For this review, take the finished solid that the model builds, in its own axes (mm). Face numbers are marked on the shaded views. Give positions to 0.01 mm unless a question says otherwise; leave off trailing zeros. Order: outer loops, then holes, each group sorted by start corner. A loop starts at its lowest first (then second) coordinate and runs counter-clockwise, first axis right, second up. Notation, with made-up numbers: M -20.5,34 L 10.5,34 A16 ccw 10.5,42 Z; hole C -2,27.5 d5. An arc over 180 degrees is marked long. Answer as CSV lines item,"result". Start each with the question number.
1. For line 1 along X through (y, z) = (10.9, 0); line 2 along X through (y, z) = (1.6, 0); line 3 along Y through (x, z) = (-49, 4.75), list the stretches that pass through material, from the lowest coordinate up.
2. Mouldability with a two-part tool opening along Y and no side actions: class the marked faces 1, 2 and 3 as pulls with the +Y half, pulls with the -Y half, needs draft (parallel to the pull), parting line crosses it, or undercut.
3. We need section B-B, the plane x = -50.5. Give the boundary of the cut face in (y, z).
4. We need section A-A, the plane x = -3. Give the boundary of the cut face in (y, z).
5. We need section C-C, the plane x = -17.5. Give the boundary of the cut face in (y, z).
6. Clearance check with flat-ended pins moving along their axes: P1, Ø5, axis at x = -26, y = 11.5, coming from the +Z side; P2, Ø1.2, axis at x = 2.5, z = 0, coming from the -Y side; P3, Ø12, axis at x = -38, y = 7, coming from the -Z side. State where each tip first meets the part, or that it passes through.
from build123d import *

# Parameters (mm, degrees)
BOSS_EXTRUDE1_DEPTH = 14.11
SKETCH2_R           = 5.95
CUT_EXTRUDE1_DEPTH  = 5.6
SKETCH3_R           = 6.9
CUT_EXTRUDE2_DEPTH  = 0.6
SKETCH4_R           = 2.5
CUT_EXTRUDE3_DEPTH  = 70.144106761
SKETCH5_R           = 0.9
CUT_EXTRUDE4_DEPTH  = 4.4
SKETCH6_R           = 6
CUT_EXTRUDE6_DEPTH  = 2.5
BOSS_EXTRUDE5_DEPTH = 0.4
BOSS_EXTRUDE6_REACH = 73.866
SKETCH13_RX         = 6
SKETCH13_RY         = 4.596266659
SKETCH14_R          = 2.5
CUT_EXTRUDE8_DEPTH  = 8


with BuildPart() as part:
    # Sketch1 → Boss-Extrude1 (new body)
    with BuildSketch(Plane(origin=(0, 0, 0), x_dir=(1, 0, 0), z_dir=(0, 1, 0))):
        with BuildLine():
            Line((-62.34882326, 5.996720639), (-1.914938962, 7.995627519))
            ThreePointArc((-1.914938962, 7.995627519), (6.349523848, 0), (-1.914938962, -7.995627519))
            Line((-1.914938962, -7.995627519), (-62.34882326, -5.996720639))
            ThreePointArc((-62.34882326, -5.996720639), (-68.150476152, 0), (-62.34882326, 5.996720639))
        make_face()
    extrude(amount=BOSS_EXTRUDE1_DEPTH)

    # Sketch2 → Cut-Extrude1 (cut)
    with BuildSketch(Plane(origin=(0, 14.11, 0), x_dir=(1, 0, 0), z_dir=(0, 1, 0))):
        with Locations(Location((-1.650476152, 0, 0), (0, 0, 270))):
            Circle(SKETCH2_R)
    extrude(amount=-CUT_EXTRUDE1_DEPTH, mode=Mode.SUBTRACT)

    # Sketch3 → Cut-Extrude2 (cut)
    with BuildSketch(Plane(origin=(0, 14.11, 0), x_dir=(1, 0, 0), z_dir=(0, 1, 0))):
        with Locations(Location((-1.650476152, 0, 0), (0, 0, 270))):
            Circle(SKETCH3_R)
    extrude(amount=-CUT_EXTRUDE2_DEPTH, mode=Mode.SUBTRACT)

    # Sketch4 → Cut-Extrude3 (cut, through all)
    with BuildSketch(Plane(origin=(0, 8.51, 0), x_dir=(1, 0, 0), z_dir=(0, 1, 0))):
        with Locations(Location((-1.650476152, 0, 0), (0, 0, 270))):
            Circle(SKETCH4_R)
    extrude(amount=-CUT_EXTRUDE3_DEPTH, mode=Mode.SUBTRACT)

    # Sketch5 → Cut-Extrude4 (cut)
    with BuildSketch(Plane(origin=(0, 8.51, 0), x_dir=(1, 0, 0), z_dir=(0, 1, 0))):
        with Locations(Location((-4.832456668, 3.181980515, 0), (0, 0, 270))):
            Circle(SKETCH5_R)
    extrude(amount=-CUT_EXTRUDE4_DEPTH, mode=Mode.SUBTRACT)

    # Sketch6 → Cut-Extrude6 (cut)
    with BuildSketch(Plane.XZ):
        with Locations(Location((-1.650476152, 0, 0), (0, 0, 270))):
            Circle(SKETCH6_R)
    extrude(amount=-CUT_EXTRUDE6_DEPTH, mode=Mode.SUBTRACT)

    # Sketch10 → Boss-Extrude5 (add)
    with BuildSketch(Plane.XZ.offset(-2.5)):
        with BuildLine():
            Line((0.75768614, -0.671382434), (4.34720185, -0.1669089))
            ThreePointArc((4.34720185, -0.1669089), (4.29113226, 0.835038606), (4.068855648, 1.813627238))
            Line((4.068855648, 1.813627238), (0.479339938, 1.309153704))
            ThreePointArc((0.479339938, 1.309153704), (0.82519402, 0.347932752), (0.75768614, -0.671382434))
        make_face()
        with BuildLine():
            Line((-7.648154155, 0.1669089), (-4.058638445, 0.671382434))
            ThreePointArc((-4.058638445, 0.671382434), (-4.126146324, -0.347932752), (-3.780292243, -1.309153704))
            Line((-3.780292243, -1.309153704), (-7.369807953, -1.813627238))
            ThreePointArc((-7.369807953, -1.813627238), (-7.592084565, -0.835038606), (-7.648154155, 0.1669089))
        make_face()
    extrude(amount=BOSS_EXTRUDE5_DEPTH)

    # Boss-Extrude6: up to this plane
    boss_extrude6_end = Plane(origin=(-1.650476152, 14.11, 0), z_dir=(0, 1, 0))
    # Sketch13 → Boss-Extrude6 (add, up to the surface)
    with BuildSketch(Plane(origin=(-0.382193209, 13.778273936, -11.555025608), x_dir=(0.9997443283307086, 0.02124917717972034, -0.007729840862870826), z_dir=(-0.02124917717972034, 0.766044443118977, -0.6424362876081342)), mode=Mode.PRIVATE) as boss_extrude6_sk1:
        with Locations(Location((-61.834760146, -9.545189308), (0, 0, -178.105579493))):
            Ellipse(SKETCH13_RX, SKETCH13_RY)
    boss_extrude6_tool1 = split(extrude(boss_extrude6_sk1.sketch, amount=-BOSS_EXTRUDE6_REACH, mode=Mode.PRIVATE), bisect_by=boss_extrude6_end, keep=Keep.BOTH, mode=Mode.PRIVATE)
    add(boss_extrude6_tool1.solids().sort_by_distance((-62.274927, 18.596512, -3.762573))[0])

    # Sketch14 → Cut-Extrude8 (cut)
    with BuildSketch(Plane(origin=(-0.382193209, 13.778273936, -11.555025608), x_dir=(0.9997742107441985, 0.01628149028495012, -0.013654325502060603), z_dir=(-0.02124917717972034, 0.766044443118977, -0.6424362876081342))):
        with Locations(Location((-62.096233495, -9.094616235, 0), (0, 0, 270))):
            Circle(SKETCH14_R)
    extrude(amount=-CUT_EXTRUDE8_DEPTH, mode=Mode.SUBTRACT)


solid = part.part
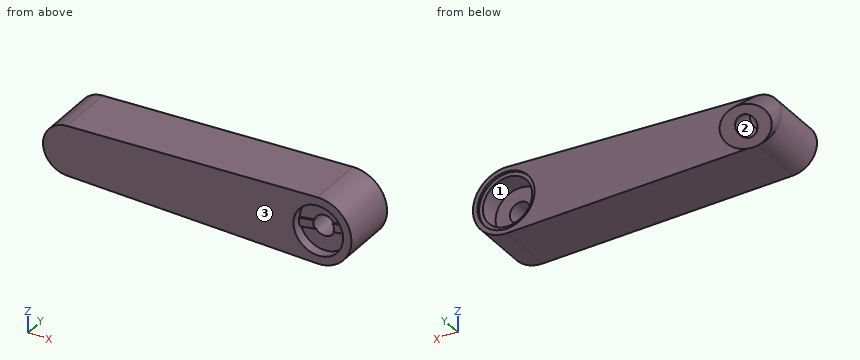
Result set:
1,line 1,"-68.15 to -7.6, 4.3 to 6.35"
1,line 2,"-68.15 to -7.65, 4.35 to 6.35"
1,line 3,"0 to 14.11"
2,face 1,"needs draft"
2,face 2,"undercut"
2,face 3,"pulls with the -Y half"
3,outline,"M 0,-6.39 L 14.11,-6.39 L 14.11,6.39 L 0,6.39 Z"
4,outline,"M 0,-7.96 L 14.11,-7.96 L 14.11,-6.77 L 13.51,-6.77 L 13.51,-5.79 L 8.51,-5.79 L 8.51,-2.1 L 2.5,-2.1 L 2.5,-5.85 L 0,-5.85 Z; M 0,5.85 L 2.5,5.85 L 2.5,2.1 L 8.51,2.1 L 8.51,5.79 L 13.51,5.79 L 13.51,6.77 L 14.11,6.77 L 14.11,7.96 L 0,7.96 Z"
5,outline,"M 0,-7.48 L 14.11,-7.48 L 14.11,7.48 L 0,7.48 Z"
6,P1,"z = 7.28"
6,P2,"y = 2.1"
6,P3,"z = -7"
